The listing builds one solid part. Answer for the finished solid, in the listing's coordinates (mm). Round coordinates to 2 decimals unless told otherwise and drop trailing zeros. Order: outer loops, then holes, each group sorted by start corner. A loop starts at its lowest first (then second) coordinate and runs counter-clockwise, first axis right, second up. Notation, with made-up numbers: M 1.5,-28.5 L 50.5,-28.5 A14 cw 50.5,-5.5 Z; hole C -19,31.25 d6. An arc over 180 degrees is marked long. Put each result on its own line as item: value. Start each with the question number.
1. Each of these flat-tipped pins is pushed along its axis until it touches: pin 1 Ø1 at (y, z) = (1, -27.5) entering from +X; pin 2 Ø1 at (x, y) = (-72, 2) entering from -Z; pin 3 Ø1.6 at (y, z) = (1.5, -26.5) entering from -X. Where does it stop, or does it pass through?
2. The part is cut by section B-B (y = 0.5). Count the separate pieces of the cut face and the enclosed holes in it, then the cut area to 3 significant figures.
3. Consider line 1 (X direction, y = 2.05, z = 26.5); line 2 (Z direction, x = 32, y = 0.7) (3 decimals); line 3 (X direction, y = 0.55, z = -13.5). Determine where each line is inside the solid, lowest interval first.
4. The part is cut by section D-D (x = 110.5). Give the vertices of the cut face in (y, z) (3 decimals).
5. The part is cut by section C-C (z = 22.5). Give the vertices of the cut face in (x, y) (3 decimals).
6. The part is cut by section A-A (x = 17.5). Give the vertices of the cut face in (y, z) (3 decimals).
from build123d import *

# Parameters (mm, degrees)
SKETCH1_W           = 25.4
SKETCH1_H           = 3.175
BOSS_EXTRUDE1_DEPTH = 3.175


with BuildPart() as part:
    # Sketch1 → Boss-Extrude1 (new body)
    with BuildSketch(Plane(origin=(0, 0, 0), x_dir=(1, 0, 0), z_dir=(0, 1, 0))):
        Polygon((-133.525, 25.4), (-133.525, 19.05), (-94.7, 19.05), (-94.7, -25.4), (-63.5, -25.4), (-63.5, -28.575), (-94.7, -28.575), (-94.7, -31.75), (94.7, -31.75), (94.7, -28.575), (63.5, -28.575), (63.5, -25.4), (94.7, -25.4), (94.7, 19.05), (133.525, 19.05), (133.525, 25.4), (63.5, 25.4), (63.5, 28.575), (38.1, 28.575), (38.1, 25.4), (12.7, 25.4), (12.7, 28.575), (-12.7, 28.575), (-12.7, 25.4), (-38.1, 25.4), (-38.1, 28.575), (-63.5, 28.575), (-63.5, 25.4), align=None)
        with Locations((25.4, -26.9875)):
            Rectangle(SKETCH1_W, SKETCH1_H, mode=Mode.SUBTRACT)
        with Locations((-25.4, -26.9875)):
            Rectangle(SKETCH1_W, SKETCH1_H, mode=Mode.SUBTRACT)
    extrude(amount=BOSS_EXTRUDE1_DEPTH)


solid = part.part
Resolved:
1. pin 1: x = 63.5
1. pin 2: z = -25.4
1. pin 3: x = -63.5
2. separate pieces: 1
2. enclosed holes: 2
2. area: 11,200 mm2
3. line 1: -63.5 to -38.1, -12.7 to 12.7, 38.1 to 63.5
3. line 2: -25.4 to 25.4, 28.575 to 31.75
3. line 3: -94.7 to 94.7
4. outline: M 0,-25.4 L 3.175,-25.4 L 3.175,-19.05 L 0,-19.05 Z
5. outline: M -94.7,0 L 94.7,0 L 94.7,3.175 L -94.7,3.175 Z
6. outline: M 0,-25.4 L 3.175,-25.4 L 3.175,25.4 L 0,25.4 Z; M 0,28.575 L 3.175,28.575 L 3.175,31.75 L 0,31.75 Z
